from build123d import *
from build123d.topology import SkipClean

# Parameters (mm, degrees)
SKETCH1_W               = 195
SKETCH1_H               = 136
SKETCH1_W_2             = 171
SKETCH1_H_2             = 112
SKETCH1_W_3             = 160
SKETCH1_H_3             = 96
SKETCH1_W_4             = 29
SKETCH1_H_4             = 3
BOSS_EXTRUDE1_DEPTH     = 2
SKETCH1_3_W             = 195
SKETCH1_3_H             = 136
SKETCH1_3_W_2           = 171
SKETCH1_3_H_2           = 112
SKETCH1_3_W_3           = 160
SKETCH1_3_H_3           = 96
SKETCH1_3_W_4           = 29
SKETCH1_3_H_4           = 3
BOSS_EXTRUDE2_DEPTH     = 2
CUT_EXTRUDE1_DEPTH      = 1.375
CUT_EXTRUDE1_DEPTH_BACK = 1.375
SKETCH2_R               = 3.25


with BuildPart() as part:
    # Sketch1 → Boss-Extrude1 (new body)
    # profile 1 of 3: a face of its own
    with BuildSketch(Plane.XY):
        Rectangle(SKETCH1_W, SKETCH1_H)
        Polygon((85.5, 56), (85.5, -56), (14.5, -56), (14.5, -59), (-14.5, -59), (-14.5, -56), (-85.5, -56), (-85.5, 56), align=None, mode=Mode.SUBTRACT)
    # profile 2 of 3: a face of its own
    with BuildSketch(Plane.XY):
        Rectangle(SKETCH1_W_2, SKETCH1_H_2)
        with Locations((0, 3)):
            Rectangle(SKETCH1_W_3, SKETCH1_H_3, mode=Mode.SUBTRACT)
    # profile 3 of 3: a face of its own
    with BuildSketch(Plane.XY):
        with Locations((0, -57.5)):
            Rectangle(SKETCH1_W_4, SKETCH1_H_4)
    extrude(amount=-BOSS_EXTRUDE1_DEPTH)

    # Sketch1_3 → Boss-Extrude2 (add)
    # profile 1 of 3: a face of its own
    with BuildSketch(Plane.XY):
        Rectangle(SKETCH1_3_W, SKETCH1_3_H)
        Polygon((85.5, 56), (85.5, -56), (14.5, -56), (14.5, -59), (-14.5, -59), (-14.5, -56), (-85.5, -56), (-85.5, 56), align=None, mode=Mode.SUBTRACT)
    # profile 2 of 3: a face of its own
    with BuildSketch(Plane.XY):
        Rectangle(SKETCH1_3_W_2, SKETCH1_3_H_2)
        with Locations((0, 3)):
            Rectangle(SKETCH1_3_W_3, SKETCH1_3_H_3, mode=Mode.SUBTRACT)
    # profile 3 of 3: a face of its own
    with BuildSketch(Plane.XY):
        with Locations((0, -57.5)):
            Rectangle(SKETCH1_3_W_4, SKETCH1_3_H_4)
    extrude(amount=BOSS_EXTRUDE2_DEPTH)

    # Sketch2 → Cut-Extrude1 (cut, two sides: drawn at the far end of the back side and taken through both)
    with SkipClean():  # the faces are left unmerged after this step: merging them gives an invalid solid
        with BuildSketch(Plane.XY.offset(-CUT_EXTRUDE1_DEPTH_BACK)):
            with Locations((-90.5, 61)):
                Circle(SKETCH2_R)
            with Locations((90.5, 61)):
                Circle(SKETCH2_R)
            with Locations((-30.166666667, -61)):
                Circle(SKETCH2_R)
            with Locations((30.166666667, -61)):
                Circle(SKETCH2_R)
            with Locations((90.5, 0)):
                Circle(SKETCH2_R)
            with Locations((-30.166666667, 61)):
                Circle(SKETCH2_R)
            with Locations((30.166666667, 61)):
                Circle(SKETCH2_R)
            with Locations((-90.5, 0)):
                Circle(SKETCH2_R)
        extrude(amount=CUT_EXTRUDE1_DEPTH + CUT_EXTRUDE1_DEPTH_BACK, mode=Mode.SUBTRACT)


solid = part.part
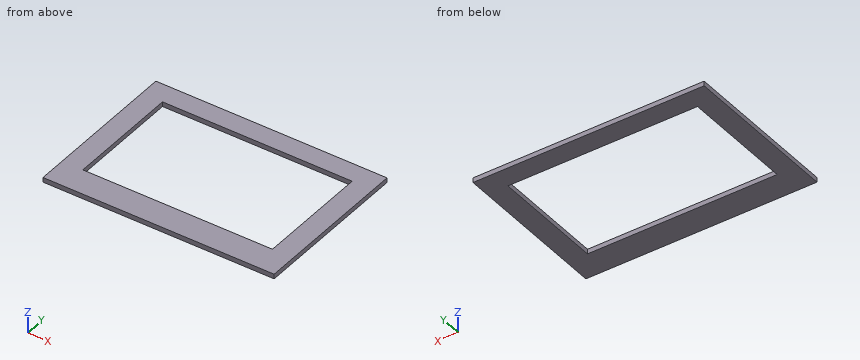
Can you work these out from the model? Positions are in its coordinate system, mm. Round coordinates to 2 decimals unless told otherwise and drop trailing zeros. Write each loop counter-clockwise with the first axis right and the second up, starting at its lowest first coordinate (ties: lowest second). Pieces come first, ordered by that corner, then holes. Notation, with made-up numbers: M -21,28 L -1,28 A17 ccw -1,56 Z; hole C -15,-1 d8. An arc over 180 degrees is marked long. Use CSV: the item, a comma, the result in double quotes.
(1) Imagine slicing it at A-A (y = 0). Write out the boundary of the cut face in (x, z) (3 decimals), plus the area to 3 significant figures.
Check values:
outline,"M -97.5,-2 L -80,-2 L -80,2 L -97.5,2 Z; M 80,-2 L 97.5,-2 L 97.5,2 L 80,2 Z; hole M -93.75,-1.375 L -87.25,-1.375 L -87.25,1.375 L -93.75,1.375 Z; hole M 87.25,-1.375 L 93.75,-1.375 L 93.75,1.375 L 87.25,1.375 Z"
area,"104 mm^2"
(2) I need wall thicknesses on line 1 along Y through (x, z) = (-90.5, 0); line 2 along Y through (x, z) = (25, -0.6); line 3 along X through (y, z) = (-37.5, 0.1). Which ranges of each line are inside material? Lowest first, please.
Check values:
line 1,"-68 to -3.25, 3.25 to 57.75, 64.25 to 68"
line 2,"-68 to -45, 51 to 68"
line 3,"-97.5 to -80, 80 to 97.5"
(3) Imagine slicing it at D-D (z = -0.6). Count the separate pieces of the cut face and the enclosed holes in it, plus the area to 3 significant figures.
Check values:
separate pieces,"1"
enclosed holes,"9"
area,"10,900 mm^2"
(4) Imagine slicing it at B-B (x = 62). Write out the boundary of the cut face in (y, z), plus the area to 3 significant figures.
Check values:
outline,"M -68,-2 L -45,-2 L -45,2 L -68,2 Z; M 51,-2 L 68,-2 L 68,2 L 51,2 Z"
area,"160 mm^2"
(5) Imagine slicing it at C-C (y = 39). Write out the boundary of the cut face in (x, z).
Check values:
outline,"M -97.5,-2 L -80,-2 L -80,2 L -97.5,2 Z; M 80,-2 L 97.5,-2 L 97.5,2 L 80,2 Z"
